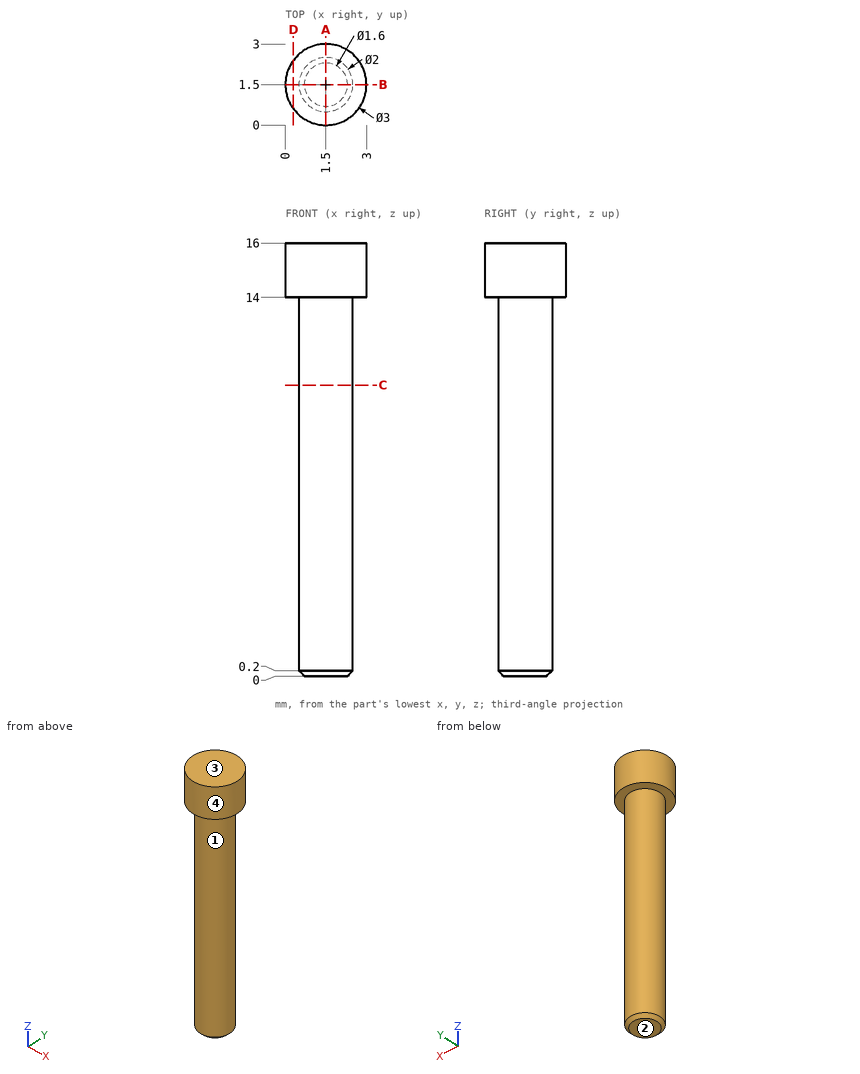
Drawing for the job (mm, zero at the part's lowest x, y, z). A direction names the side the tool comes from. Coordinates: 2 decimals unless noted, no trailing zeros. Order: outer loops, then holes, each group sorted by start corner. A loop starts at its lowest first (then second) coordinate and runs counter-clockwise, first axis right, second up. Notation, with made-up numbers: (-9.5, 53.25) - (23.5, 53.25) arc R14 ccw to (23.5, 75.25) - close; hole circle Ø11 at (83.25, 52). An arc over 180 degrees is marked (long way). Use a Markdown table: item, result. Add a question column.
(1) Saw through at A-A (x = 1.5). Give the cut face in (y, z), then the cut area to 3 significant figures.
(2) Flat gauge pins, fed straight in: pin 1 (0.9 mm diameter, centred on x = 1.5, y = 1, fed in from -Z); pin 2 (1.5 mm diameter, centred on y = 0.5, z = 3, fed in from +X). Where does each tip first touch, or does it go through?
(3) Saw through at C-C (z = 10.75). Give the cut face in (x, y).
(4) Saw through at D-D (x = 0.3). Give the cut face in (y, z), then the cut area to 3 significant figures.
(5) Which spindle directions (+Z, -Z, +X, -X, +Y, -Y) get a long thin tool onto all of the face, cutting with end or side? Do the marked faces 1 and 2. Say none if no direction does.
(6) Drill centre lines: line 1 along Z through (x, y) = (2.55, 1); line 2 along X through (y, z) = (1.1, 11.25); line 3 along X through (y, z) = (0.75, 13.25). Where is each one in solid material? Low to high. Write a range as [from, to].
(7) Pull direction Y, two halves, no side cores. Call the marked faces 3 and 4: +Y half, -Y half, draft (parallel to the pull), parting line (faces both ways), or undercut.
Solved:
| question | item | result |
|---|---|---|
| 1 | outline | (0, 14) - (0.5, 14) - (0.5, 0.2) - (0.7, 0) - (2.3, 0) - (2.5, 0.2) - (2.5, 14) - (3, 14) - (3, 16) - (0, 16) - close |
| 1 | area | 34.0 mm² |
| 2 | pin 1 | stops at z = 0 |
| 2 | pin 2 | stops at x = 2.47 |
| 3 | outline | circle Ø2 at (1.5, 1.5) |
| 4 | outline | (0.6, 14) - (2.4, 14) - (2.4, 16) - (0.6, 16) - close |
| 4 | area | 3.60 mm² |
| 5 | face 1 | -Z |
| 5 | face 2 | -Z, +X, -X, +Y, -Y |
| 6 | line 1 | z = [14, 16] |
| 6 | line 2 | x = [0.58, 2.42] |
| 6 | line 3 | x = [0.84, 2.16] |
| 7 | face 3 | draft |
| 7 | face 4 | parting line |
